Work out the finished part from the listing and answer in its coordinate system (mm). Face numbers are marked on the shaded views. A direction names the side the tool comes from. Give positions to 0.01 mm unless a question says otherwise; leave off trailing zeros. Order: outer loops, then holes, each group sorted by start corner. A loop starts at its lowest first (then second) coordinate and runs counter-clockwise, first axis right, second up. Notation, with made-up numbers: (47.5, 73.5) - (51.5, 73.5) arc R16 ccw to (51.5, 77.5) - close; hole circle Ø5 at (-20.75, -5). An arc over 180 degrees is marked (long way). Write each question's results on one line, items separated by ' | '.
from build123d import *

# Parameters (mm, degrees)
SKETCH1_R           = 1.5
BOSS_EXTRUDE1_DEPTH = 2.5
BOSS_EXTRUDE2_START = -2.5
SKETCH2_R           = 18
BOSS_EXTRUDE2_DEPTH = 17
SKETCH3_R           = 8
BOSS_EXTRUDE3_DEPTH = 1.8
SKETCH4_R           = 2.5
BOSS_EXTRUDE4_DEPTH = 5


with BuildPart() as part:
    # Sketch1 → Boss-Extrude1 (new body)
    with BuildSketch(Plane(origin=(0, 0, 0), x_dir=(1, 0, 0), z_dir=(0, 1, 0))):
        with BuildLine():
            Line((-16.237503877, 7.768105807), (-23.86592771, 2.961133868))
            ThreePointArc((-23.86592771, 2.961133868), (-25.5, 0), (-23.86592771, -2.961133868))
            Line((-23.86592771, -2.961133868), (-16.237503877, -7.768105807))
            ThreePointArc((-16.237503877, -7.768105807), (0, -18), (16.237503877, -7.768105807))
            Line((16.237503877, -7.768105807), (23.86592771, -2.961133868))
            ThreePointArc((23.86592771, -2.961133868), (25.5, 0), (23.86592771, 2.961133868))
            Line((23.86592771, 2.961133868), (16.237503877, 7.768105807))
            ThreePointArc((16.237503877, 7.768105807), (0, 18), (-16.237503877, 7.768105807))
        make_face()
        with Locations(Location((-22, 0, 0), (0, 0, 270))):
            Circle(SKETCH1_R, mode=Mode.SUBTRACT)
        with Locations(Location((22, 0, 0), (0, 0, 90))):
            Circle(SKETCH1_R, mode=Mode.SUBTRACT)
    extrude(amount=BOSS_EXTRUDE1_DEPTH)

    # Sketch2 → Boss-Extrude2 (add)
    with BuildSketch(Plane(origin=(0, 2.5, 0), x_dir=(1, 0, 0), z_dir=(0, 1, 0)).offset(BOSS_EXTRUDE2_START)):
        with Locations(Location((0, 0, 0), (0, 0, 25.566693529))):
            Circle(SKETCH2_R)
    extrude(amount=BOSS_EXTRUDE2_DEPTH)

    # Sketch3 → Boss-Extrude3 (add)
    with BuildSketch(Plane.XZ):
        with Locations(Location((0, 0, 0), (0, 0, 270))):
            Circle(SKETCH3_R)
    extrude(amount=BOSS_EXTRUDE3_DEPTH)

    # Sketch4 → Boss-Extrude4 (add)
    with BuildSketch(Plane.XZ.offset(1.8)):
        with Locations(Location((0, 0, 0), (0, 0, 270))):
            Circle(SKETCH4_R)
    extrude(amount=BOSS_EXTRUDE4_DEPTH)


solid = part.part
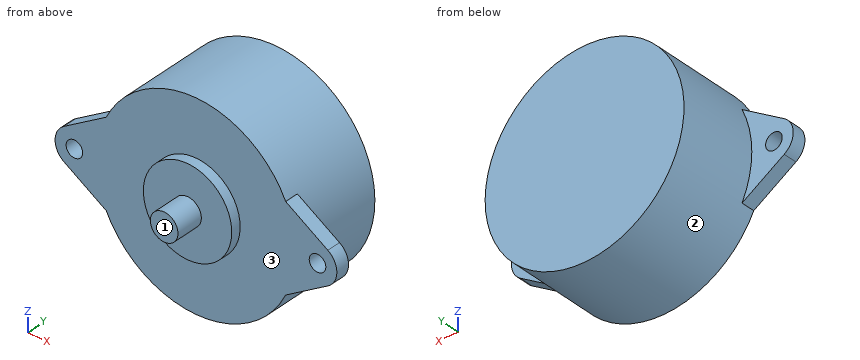
1. A cutting plane is placed at C-C, the plane x = -22. Write down the section's boundary in (y, z).
Answer list:
outline: (0, -4.14) - (2.5, -4.14) - (2.5, -1.5) - (0, -1.5) - close; (0, 1.5) - (2.5, 1.5) - (2.5, 4.14) - (0, 4.14) - close
2. Straight lines are drawn through the part: line 1 (X direction, y = 1.5, z = -0.5); line 2 (Y direction, x = 10, z = -0.5); line 3 (Y direction, x = 5, z = 4). For each, find the intervals that lie inside material, in ascending order. Write a range as [from, to].
Answer list:
line 1: [-25.46, -23.41], [-20.59, 20.59], [23.41, 25.46] | line 2: [0, 17] | line 3: [-1.8, 17]
3. Given P1, Ø1, axis at x = 11, z = 1, coming from the -Y side; P2, Ø5, axis at x = 10, y = -2, coming from the +Z side; P3, Ø7.5, axis at x = 20.5, z = 1.5, coming from the +Y side; P4, Ø1.5, axis at y = 9, z = -10, coming from the +X side, each flat-ended and moving along its own axis, determine where each tip first touches the part or whether it passes through.
Answer list:
P1: y = 0 | P2: z = 15.87 | P3: y = 17 | P4: x = 15.44
4. A tool of negligible diameter and unlimited length cuts with its end or side. For the marked faces 1, 2 and 3, from which of +Z, -Z, +X, -X, +Y, -Y can it reach the whole face along a straight path? Write none if from no direction.
Answer list:
face 1: +Z, -Z, +X, -X, -Y | face 2: +Y | face 3: -Y
5. A cutting plane is placed at A-A, the plane z = 0. Write down the section's boundary in (x, y).
Answer list:
outline: (-25.5, 0) - (-23.5, 0) - (-23.5, 2.5) - (-25.5, 2.5) - close; (-20.5, 0) - (-8, 0) - (-8, -1.8) - (-2.5, -1.8) - (-2.5, -6.8) - (2.5, -6.8) - (2.5, -1.8) - (8, -1.8) - (8, 0) - (20.5, 0) - (20.5, 2.5) - (18, 2.5) - (18, 17) - (-18, 17) - (-18, 2.5) - (-20.5, 2.5) - close; (23.5, 0) - (25.5, 0) - (25.5, 2.5) - (23.5, 2.5) - close
6. A cutting plane is placed at D-D, the plane x = 0. Write down the section's boundary in (y, z), then the cut area to 3 significant figures.
Answer list:
outline: (-6.8, -2.5) - (-1.8, -2.5) - (-1.8, -8) - (0, -8) - (0, -18) - (17, -18) - (17, 18) - (0, 18) - (0, 8) - (-1.8, 8) - (-1.8, 2.5) - (-6.8, 2.5) - close | area: 666 mm^2
7. A cutting plane is placed at B-B, the plane y = 0.75. Write down the section's boundary in (x, z).
Answer list:
outline: (-23.87, -2.96) - (-16.24, -7.77) arc R18 ccw to (16.24, -7.77) - (23.87, -2.96) arc R3.5 ccw to (23.87, 2.96) - (16.24, 7.77) arc R18 ccw to (-16.24, 7.77) - (-23.87, 2.96) arc R3.5 ccw to start; hole circle Ø3 at (-22, 0); hole circle Ø3 at (22, 0)
